For this review, take the finished solid that the model builds, in its own axes (mm). A direction names the side the tool comes from. Coordinates: 2 decimals unless noted, no trailing zeros. Loops run counter-clockwise (first coordinate to the right, second up) from the corner with the lowest first, then second, coordinate; pieces in that order, holes last. Notation, with made-up numbers: (1.5, 54.25) -> (37.5, 54.25) arc R12 ccw to (37.5, 64.25) -> close; hole circle Ø6 at (78, -26.75). An arc over 180 degrees is marked (long way). Answer in a Markdown table with one row per item.
from build123d import *

# Parameters (mm, degrees)
F1_DEPTH = 30
F2_W     = 3
F2_H     = 25
F2_W_2   = 47
F2_H_2   = 27
F3_DEPTH = 14.001
F4_D     = 4.4
F6_D     = 3.3
F7_R     = 3


with BuildPart() as f1:
    # F0 (on Top) → F1 (new body, symmetric)
    with BuildSketch(Plane.XY):
        with BuildLine():
            Line((-52.5, 0), (52.5, 0))
            ThreePointArc((52.5, 0), (53.2071067812, -0.2928932188), (53.5, -1))
            Line((53.5, -1), (53.5, -12))
            Line((53.5, -12), (55.5, -12))
            Line((55.5, -12), (55.5, -1))
            ThreePointArc((55.5, -1), (54.6213203436, 1.1213203436), (52.5, 2))
            Line((52.5, 2), (-52.5, 2))
            ThreePointArc((-52.5, 2), (-54.6213203436, 1.1213203436), (-55.5, -1))
            Line((-55.5, -1), (-55.5, -12))
            Line((-55.5, -12), (-53.5, -12))
            Line((-53.5, -12), (-53.5, -1))
            ThreePointArc((-53.5, -1), (-53.2071067812, -0.2928932188), (-52.5, 0))
        make_face()
    extrude(amount=F1_DEPTH, both=True)

    # F2 (on face) → F3 (cut, through all)
    with BuildSketch(Plane(origin=(0, 2, 0), x_dir=(-1, 0, 0), z_dir=(0, 1, 0))):
        with Locations((-54, 0)):
            Rectangle(F2_W, F2_H)
        with Locations((54, 0)):
            Rectangle(F2_W, F2_H)
        Rectangle(F2_W_2, F2_H_2)
    extrude(amount=-F3_DEPTH, mode=Mode.SUBTRACT)

    # F4 (through all)
    with Locations(Plane(origin=(0, 2, 0), x_dir=(-1, 0, 0), z_dir=(0, 1, 0))):
        with Locations((0, 20), (0, -20)):
            Hole(F4_D / 2)

    # F6 (through all)
    with Locations(Plane.YZ.offset(55.5)):
        with Locations((-6.5, 21.25), (-6.5, -21.25)):
            Hole(F6_D / 2)

    # F7
    f7_edges = [f1.edges().sort_by_distance(p)[0] for p in [
        (-54.5, -12, 30),
        (-54.5, -12, 12.5),
        (-54.5, -12, -12.5),
        (-54.5, -12, -30),
        (54.5, -12, 30),
        (54.5, -12, 12.5),
        (54.5, -12, -12.5),
        (54.5, -12, -30),
    ]]
    fillet(f7_edges, radius=F7_R)


solid = f1.part
Item 1: Take a section at A-A, the plane y = -2.25. State the section outline as (x, z) points, and give its area (3 significant figures).
Worked answers:
| item | result |
|---|---|
| outline | (-55.5, -30) -> (-53.5, -30) -> (-53.5, -12.5) -> (-55.5, -12.5) -> close; (-55.5, 12.5) -> (-53.5, 12.5) -> (-53.5, 30) -> (-55.5, 30) -> close; (53.5, -30) -> (55.5, -30) -> (55.5, -12.5) -> (53.5, -12.5) -> close; (53.5, 12.5) -> (55.5, 12.5) -> (55.5, 30) -> (53.5, 30) -> close |
| area | 140 mm² |
Item 2: Take a section at B-B, the plane x = -10. State the section outline as (y, z) points, and give its area (3 significant figures).
Worked answers:
| item | result |
|---|---|
| outline | (0, -30) -> (2, -30) -> (2, -13.5) -> (0, -13.5) -> close; (0, 13.5) -> (2, 13.5) -> (2, 30) -> (0, 30) -> close |
| area | 66.0 mm² |
Item 3: For L1, parallel to Z at x = 0, y = 0.9; L2, parallel to Z at x = 55.15, y = -6.5; L3, parallel to X at y = -5.75, z = -14.5, list the stretches that pass through material, from the lowest coordinate up.
Worked answers:
| item | result |
|---|---|
| L1 | -30 to -22.2, -17.8 to -13.5, 13.5 to 17.8, 22.2 to 30 |
| L2 | -30 to -22.9, -19.6 to -12.5, 12.5 to 19.6, 22.9 to 30 |
| L3 | -55.5 to -53.5, 53.5 to 55.5 |
Item 4: Take a section at D-D, the plane z = -25.5. State the section outline as (x, y) points, and give its area (3 significant figures).
Worked answers:
| item | result |
|---|---|
| outline | (-55.5, -12) -> (-53.5, -12) -> (-53.5, -1) arc R1 cw to (-52.5, 0) -> (52.5, 0) arc R1 cw to (53.5, -1) -> (53.5, -12) -> (55.5, -12) -> (55.5, -1) arc R3 ccw to (52.5, 2) -> (-52.5, 2) arc R3 ccw to (-55.5, -1) -> close |
| area | 267 mm² |
Item 5: The part is to be moulded in two halves that separate along Z. For faces 4 (the cylindrical face through (-54.49, -11.1, -29.14)), 5 (the cylindrical face through (-54.49, -11.14, -13.4)), 6 (the flat face through (54, -12, -21)), say which applies: +Z half, -Z half, draft (parallel to the pull), parting line (faces both ways), or undercut.
Worked answers:
| item | result |
|---|---|
| face 4 | -Z half |
| face 5 | undercut |
| face 6 | draft |
Item 6: Take a section at C-C, the plane z = 0. State the section outline as (x, y) points, and give its area (3 significant figures).
Worked answers:
| item | result |
|---|---|
| outline | (-52.5, 0) -> (-23.5, 0) -> (-23.5, 2) -> (-52.5, 2) -> close; (23.5, 0) -> (52.5, 0) -> (52.5, 2) -> (23.5, 2) -> close |
| area | 116 mm² |
Item 7: For faces 1 (the flat face through (53.5, -6, 19)), 2 (the flat face through (0, 1, 13.5)), 3 (the cylindrical face through (-54.49, -11.1, 13.36)), list the 3-axis set-ups (+Z, -Z, +X, -X, +Y, -Y) from which the entire face can be reached by the end or side of a thin tool; tool diameter is ignored.
Worked answers:
| item | result |
|---|---|
| face 1 | +Z, -Z, -Y |
| face 2 | +Y, -Y |
| face 3 | +X, -X, -Y |
Item 8: Insertion check: pin 1 (2 mm diameter, centred on y = 0.5, z = -4.5, fed in from -X); pin 2 (1 mm diameter, centred on x = 21, y = -1.5, fed in from +Z); pin 3 (5.5 mm diameter, centred on y = -6.5, z = -21.25, fed in from -X); pin 4 (2 mm diameter, centred on y = 0.5, z = 2, fed in from +X). Each pin has a flat end and moves straight along its axis. Give the tip position at first contact, or say it passes through.
Worked answers:
| item | result |
|---|---|
| pin 1 | x = -52.5 |
| pin 2 | through |
| pin 3 | x = -55.5 |
| pin 4 | x = 52.5 |
